```python
from build123d import *

# Parameters (mm, degrees)
KEEPOUTLAYER_W       = 186.9999816
KEEPOUTLAYER_H       = 76.9999984
EXTRUDE_1_DEPTH      = 1.6
VIAHOLELAYER_R       = 0.7499985
CUT_EXTRUDE_1_DEPTH  = 203.32893066
EXTRUDE_2_DEPTH      = 7.8
EXTRUDE_2_DEPTH_BACK = 9.6
SKETCH_1_W           = 15
SKETCH_1_H           = 60.9999984
SKETCH_2_W           = 5
SKETCH_2_H           = 1.6
EXTRUDE_3_DEPTH      = 2.5
SKETCH_4_W           = 7.5
SKETCH_4_H           = 8
EXTRUDE_4_DEPTH      = 16.5


with BuildPart() as part:
    # KeepOutLayer → Бобышка-Вытянуть1 (new body)
    with BuildSketch(Plane.XY):
        with Locations((93.56941662, -38.56797722)):
            Rectangle(KEEPOUTLAYER_W, KEEPOUTLAYER_H)
    extrude(amount=-EXTRUDE_1_DEPTH)

    # ViaHoleLayer → Вырез-Вытянуть1 (cut, through all)
    with BuildSketch(Plane.XY):
        with Locations((3.0693995, -73.06799966)):
            Circle(VIAHOLELAYER_R)
        with Locations((3.0693995, -4.0680005)):
            Circle(VIAHOLELAYER_R)
        with Locations((184.06940072, -73.06799966)):
            Circle(VIAHOLELAYER_R)
        with Locations((184.06940072, -4.0680005)):
            Circle(VIAHOLELAYER_R)
    extrude(amount=-CUT_EXTRUDE_1_DEPTH, mode=Mode.SUBTRACT)

    # Эскиз1 → Бобышка-Вытянуть2 (add, two sides: drawn at the far end of the back side and taken through both)
    with BuildSketch(Plane.XY.offset(-EXTRUDE_2_DEPTH_BACK)):
        with Locations((5.86942582, -38.56797722)):
            Rectangle(SKETCH_1_W, SKETCH_1_H)
    extrude(amount=EXTRUDE_2_DEPTH + EXTRUDE_2_DEPTH_BACK)

    # Эскиз2 → Бобышка-Вытянуть3 (add)
    with BuildSketch(Plane(origin=(0, -0.06797802, 0), x_dir=(1, 0, 0), z_dir=(0, 1, 0))):
        with Locations((52.56942582, 0.8)):
            Rectangle(SKETCH_2_W, SKETCH_2_H)
    extrude(amount=EXTRUDE_3_DEPTH)

    # Эскиз4 → Бобышка-Вытянуть4 (add)
    with BuildSketch(Plane(origin=(0, 0, -1.6), x_dir=(-1, 0, 0), z_dir=(0, 0, -1))):
        with Locations((-178.31940742, -74.66797642)):
            Rectangle(SKETCH_4_W, SKETCH_4_H)
    extrude(amount=EXTRUDE_4_DEPTH)


solid = part.part
```
Verification items for the finished model (mm, model axes). A direction names the side the tool comes from. Coordinates: 2 decimals unless noted, no trailing zeros. Write each loop counter-clockwise with the first axis right and the second up, starting at its lowest first coordinate (ties: lowest second). Pieces come first, ordered by that corner, then holes. Notation, with made-up numbers: M -9,-30 L 27,-30 A27 ccw 27,-9 Z; hole C 66,-22.75 d1. An arc over 180 degrees is marked long. One line per item, written item: value.
Item 1: Section check D-D, the plane z = -14.25. Record the boundary of the cut face in (x, y).
Check sheet entries:
outline: M 174.57,-78.67 L 182.07,-78.67 L 182.07,-70.67 L 174.57,-70.67 Z
Item 2: Scan lines: line 1 along Z through (x, y) = (28.5, -18.5); line 2 along X through (y, z) = (-55, -8.25); line 3 along X through (y, z) = (-2.5, -0.75). Record each from-to range of solid material in increasing order.
Check sheet entries:
line 1: z = -1.6 to 0
line 2: x = -1.63 to 13.37
line 3: x = 0.07 to 187.07
Item 3: Access from +Z, -Z, +X, -X, +Y, -Y to the whole of each face (thin tool, end or side, straight path). Record for faces 1 (the flat face through (174.569, -75, -10)), 2 (the flat face through (182.069, -75, -10)), 3 (the flat face through (178, -70.668, -10)).
Check sheet entries:
face 1: -Z, -X, +Y, -Y
face 2: -Z, +X, +Y, -Y
face 3: -Z, +X, -X, +Y
Item 4: Section check C-C, the plane x = 119. Record the boundary of the cut face in (y, z).
Check sheet entries:
outline: M -77.07,-1.6 L -0.07,-1.6 L -0.07,0 L -77.07,0 Z
Item 5: Gauge pin test, flat ends, axial feed: pin 1 Ø4 at (x, y) = (29.5, -29) entering from -Z; pin 2 Ø4.5 at (x, z) = (9, 2) entering from +Y; pin 3 Ø0.5 at (x, y) = (177.5, -77.5) entering from +Z. Record the tip position at first contact, or that the pin passes through.
Check sheet entries:
pin 1: stops at z = -1.6
pin 2: stops at y = -0.07
pin 3: stops at z = -1.6
Item 6: Section check B-B, the plane y = -61.5. Record the boundary of the cut face in (x, z).
Check sheet entries:
outline: M -1.63,-9.6 L 13.37,-9.6 L 13.37,-1.6 L 187.07,-1.6 L 187.07,0 L 13.37,0 L 13.37,7.8 L -1.63,7.8 Z
Item 7: Section check A-A, the plane z = -7. Record the boundary of the cut face in (x, y), plus the area to 3 significant figures.
Check sheet entries:
outline: M -1.63,-69.07 L 13.37,-69.07 L 13.37,-8.07 L -1.63,-8.07 Z; M 174.57,-78.67 L 182.07,-78.67 L 182.07,-70.67 L 174.57,-70.67 Z
area: 975 mm^2
